Here's how the part is built. I have some questions about the finished solid (model axes, mm). Face numbers are marked on the shaded views. A direction names the side the tool comes from. Give positions to 0.01 mm unless a question says otherwise; leave off trailing zeros. Order: outer loops, then holes, each group sorted by start corner. A loop starts at its lowest first (then second) coordinate and runs counter-clockwise, first axis right, second up. Notation, with made-up numbers: M 88.5,-30 L 140.5,-30 A27 ccw 140.5,-4 Z; hole C -37,43.5 d5. An arc over 180 degrees is marked long. Use CSV: the item, a comma, the result in double quotes. Start each with the question number.
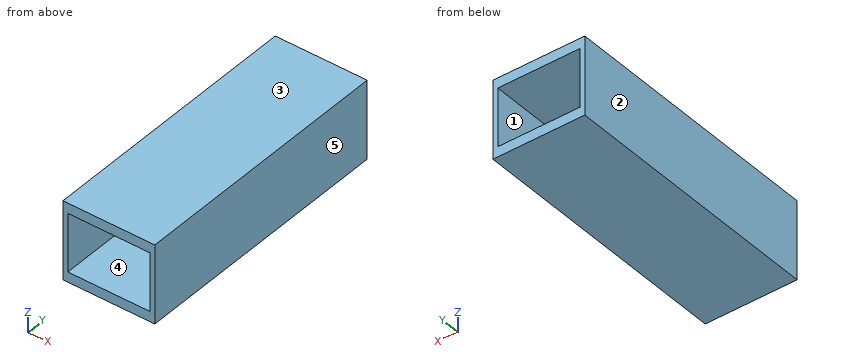
```python
from build123d import *

# Parameters (mm, degrees)
F0_W     = 304.8
F0_H     = 88.646
F1_DEPTH = 103.886
F3_W     = 92.71
F3_H     = 65.786
F4_DEPTH = 1270


with BuildPart() as f1:
    # F0 (on Right) → F1 (new body)
    with BuildSketch(Plane.YZ):
        Rectangle(F0_W, F0_H)
    extrude(amount=F1_DEPTH)

    # F3 (on face) → F4 (cut)
    with BuildSketch(Plane.XZ.offset(152.4)):
        with Locations((51.943, 0)):
            Rectangle(F3_W, F3_H)
    extrude(amount=-F4_DEPTH, mode=Mode.SUBTRACT)


solid = f1.part
```
Q1. Imagine slicing it at B-B, the plane x = 56. Please give me the cut outline in (y, z).
Q2. We'd pull the mould along X, two halves only. Please class the marked faces 3, 4 and 5: pulls with the +X half, pulls with the -X half, needs draft (parallel to the pull), parting line crosses it, or undercut.
Q3. Imagine slicing it at A-A, the plane z = -12. Please give me the cut outline in (x, y).
Q4. For P1, Ø10, axis at y = 117, z = 11, coming from the -X side, with a flat end and sliding along its axis, tell me the tip position at first contact or that it passes through.
Q5. Imagine slicing it at C-C, the plane y = -19. Please give me the cut outline in (x, z), then the cut area to 3 significant figures.
Q6. I need wall thicknesses on line 1 (Z direction, x = 7, y = 108.5); line 2 (X direction, y = 76, z = -11). Which ranges of each line are inside material? Lowest first, please. Write a range as [from, to].
Q7. For the marked faces 1 and 2, which set-ups out of +Z, -Z, +X, -X, +Y, -Y let a thin tool reach every point of the face, with its end or its side?
Reply:
1,outline,"M -152.4,-44.32 L 152.4,-44.32 L 152.4,-32.89 L -152.4,-32.89 Z; M -152.4,32.89 L 152.4,32.89 L 152.4,44.32 L -152.4,44.32 Z"
2,face 3,"needs draft"
2,face 4,"undercut"
2,face 5,"pulls with the +X half"
3,outline,"M 0,-152.4 L 5.59,-152.4 L 5.59,152.4 L 0,152.4 Z; M 98.3,-152.4 L 103.89,-152.4 L 103.89,152.4 L 98.3,152.4 Z"
4,P1,"stops at x = 0"
5,outline,"M 0,-44.32 L 103.89,-44.32 L 103.89,44.32 L 0,44.32 Z; hole M 5.59,-32.89 L 98.3,-32.89 L 98.3,32.89 L 5.59,32.89 Z"
5,area,"3,110 mm^2"
6,line 1,"z = [-44.32, -32.89], [32.89, 44.32]"
6,line 2,"x = [0, 5.59], [98.3, 103.89]"
7,face 1,"+Y, -Y"
7,face 2,"+Z, -Z, -X, +Y, -Y"
